Read the model definition and answer for the solid it produces. Units are mm, in the model's axes. Face numbers are marked on the shaded views. A direction names the side the tool comes from. Give positions to 0.01 mm unless a question says otherwise; leave off trailing zeros. Order: outer loops, then holes, each group sorted by start corner. A loop starts at its lowest first (then second) coordinate and runs counter-clockwise, first axis right, second up.
Item 1: A cutting plane is placed at D-D (x = -9.5). Write down the section's boundary in (y, z), plus the area to 3 significant figures.
Item 2: A cutting plane is placed at A-A (y = 7). Write down the section's boundary in (x, z), plus the area to 3 significant figures.
Item 3: A cutting plane is placed at B-B (z = -47). Write down the section's boundary in (x, y).
Item 4: Given pin 1 Ø6 at (x, z) = (2, 39) entering from +Y; pin 2 Ø5 at (x, y) = (8, -4) entering from +Z; pin 3 Ø12 at (y, z) = (22, 57.5) entering from +X, each flat-ended and moving along its own axis, determine where each tip first touches the part or whether it passes through.
Item 5: Which of the six approach directions +Z, -Z, +X, -X, +Y, -Y give full straight-line access (tool end or side, diameter ignored) to the marked faces 1 and 2?
Item 6: A cutting plane is placed at C-C (x = 7.75). Write down the section's boundary in (y, z), plus the area to 3 significant figures.
Item 7: Find the intervals of material crossed by line 1 along X through (y, z) = (7.5, -45); line 2 along X through (y, z) = (11.5, 4); line 3 along X through (y, z) = (34, 10.5), in increasing order.
from build123d import *

# Parameters (mm, degrees)
F1_DEPTH = 100


with BuildPart() as f1:
    # F0 (on Top) → F1 (new body, symmetric)
    with BuildSketch(Plane.XY):
        with BuildLine():
            Line((15, -8.853287), (-0.05791, 41.146713))
            Line((-0.05791, 41.146713), (-15, -8.660254))
            Line((-15, -8.660254), (-13.563261, -9.091276))
            Line((-13.563261, -9.091276), (-1.967105, 29.562577))
            ThreePointArc((-1.967105, 29.562577), (-0.052514, 30.987881), (1.863589, 29.564611))
            Line((1.863589, 29.564611), (13.56326, -9.284309))
            Line((13.56326, -9.284309), (15, -8.853287))
        make_face()
    extrude(amount=F1_DEPTH, both=True)


solid = f1.part
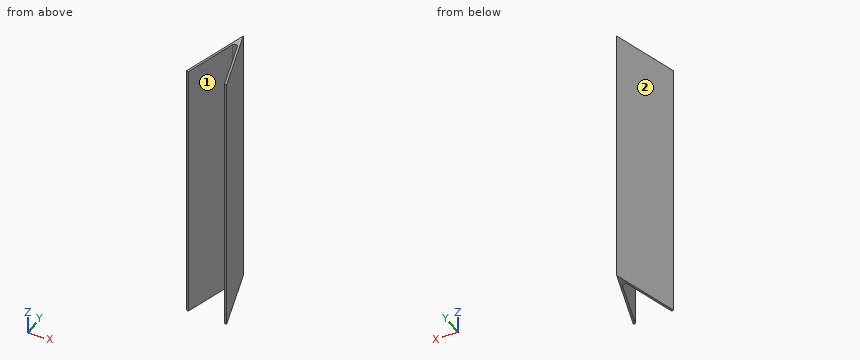
Response values:
1. outline: (4.45, -100) - (9.67, -100) - (9.67, 100) - (4.45, 100) - close
1. area: 1,040 mm2
2. outline: (-10.3, -100) - (-8.74, -100) - (-8.74, 100) - (-10.3, 100) - close; (8.66, -100) - (10.23, -100) - (10.23, 100) - (8.66, 100) - close
2. area: 627 mm2
3. outline: (-15, -8.66) - (-13.56, -9.09) - (-1.97, 29.56) arc R2 cw to (1.86, 29.56) - (13.56, -9.28) - (15, -8.85) - (-0.06, 41.15) - close
4. pin 1: stops at y = 41.15
4. pin 2: passes through
4. pin 3: stops at x = 7.52
5. face 1: +Z, -Z, -Y
5. face 2: +Z, -Z, -X, +Y
6. outline: (10.02, -100) - (15.22, -100) - (15.22, 100) - (10.02, 100) - close
6. area: 1,040 mm2
7. line 1: x = -10.15 to -8.59, 8.51 to 10.08
7. line 2: x = -8.95 to -7.39, 7.3 to 8.87
7. line 3: x = -2.2 to 2.09
